Answer from the drawing. Dimensions are ordinates in mm from the lowest x, y and z of the part. A direction names the side the tool comes from. Give positions to 0.01 mm unless a question says otherwise; leave off trailing zeros. Loops run counter-clockwise (first coordinate to the right, second up) from the corner with the lowest first, then second, coordinate; pieces in that order, holes last.
(1) Each of these flat-tipped pins is pushed along its axis until it touches: P1, Ø4, axis at x = 43.5, z = 11.5, coming from the +Y side; P2, Ø5.5, axis at x = 30.5, z = 74.5, coming from the -Y side (3 decimals); P3, Ø5, axis at x = 28.5, y = 22, coming from the -Z side. Where does it stop, or does it pass through?
(2) Find section D-D, the plane y = 32. Write down the section's boundary in (x, z), then the cut area to 3 significant figures.
(3) Find section C-C, the plane x = 46.5. Write down the section's boundary in (y, z) (3 decimals).
(4) Determine the mould class of the marked faces 4, 5, 6 and 7 for opening direction Z: pulls with the +Z half, pulls with the -Z half, needs draft (parallel to the pull), parting line crosses it, or undercut.
(5) Which of the six approach directions +Z, -Z, +X, -X, +Y, -Y give full straight-line access (tool end or side, diameter ignored) to the marked faces 1, 2 and 3?
(6) Find section A-A, the plane y = 10. Write down the section's boundary in (x, z).
(7) Find section B-B, the plane z = 17. Write down the section's boundary in (x, y), then the cut area to 3 significant figures.
(8) Straight lines are drawn through the part: probe 1 along Z at (x, y) = (48.5, 12); probe 2 along Z at (x, y) = (14, 10.5); probe 3 along Y at (x, z) = (30, 67) (3 decimals). For each, find the intervals that lie inside material, in ascending order.
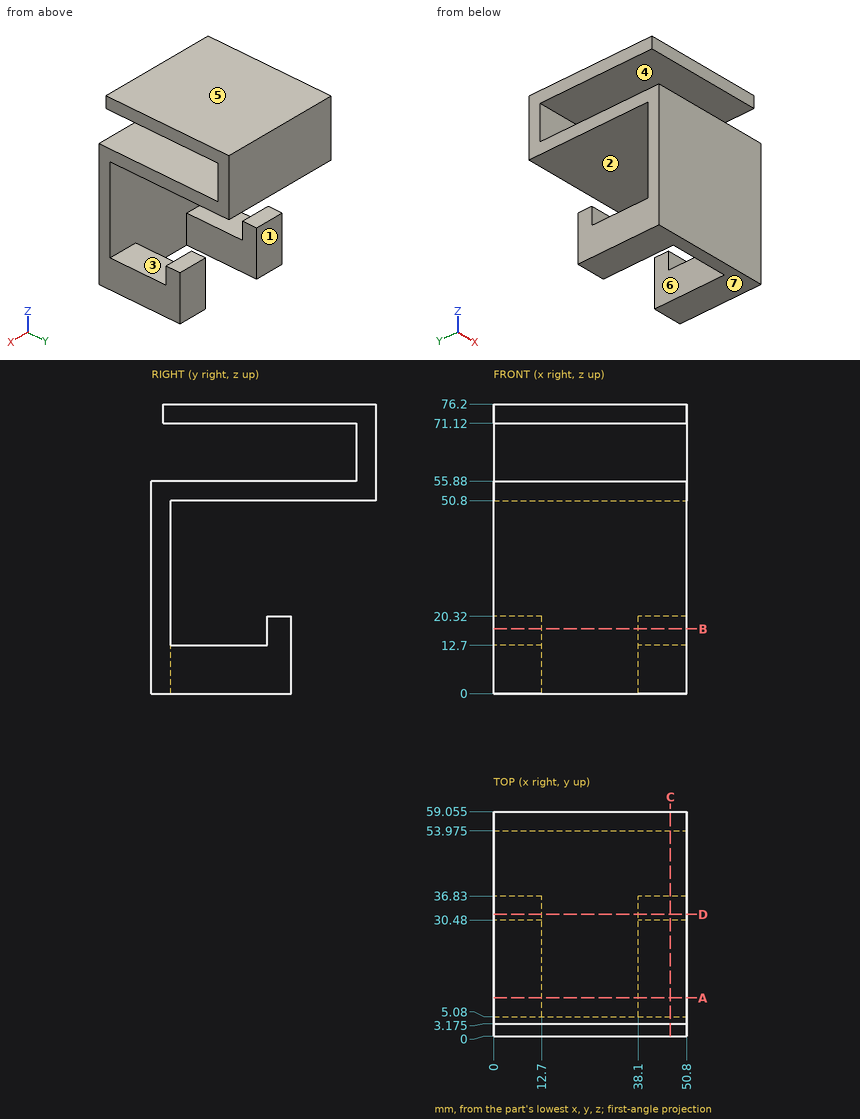
Entries:
1. P1: stops at y = 36.83
1. P2: stops at y = 3.175
1. P3: stops at z = 50.8
2. outline: (0, 0) - (12.7, 0) - (12.7, 20.32) - (0, 20.32) - close; (0, 50.8) - (50.8, 50.8) - (50.8, 55.88) - (0, 55.88) - close; (0, 71.12) - (50.8, 71.12) - (50.8, 76.2) - (0, 76.2) - close; (38.1, 0) - (50.8, 0) - (50.8, 20.32) - (38.1, 20.32) - close
2. area: 1,030 mm2
3. outline: (0, 0) - (36.83, 0) - (36.83, 20.32) - (30.48, 20.32) - (30.48, 12.7) - (5.08, 12.7) - (5.08, 50.8) - (59.055, 50.8) - (59.055, 76.2) - (3.175, 76.2) - (3.175, 71.12) - (53.975, 71.12) - (53.975, 55.88) - (0, 55.88) - close
4. face 4: undercut
4. face 5: pulls with the +Z half
4. face 6: needs draft
4. face 7: pulls with the -Z half
5. face 1: -Z, +X, -X, +Y
5. face 2: +X, -X, +Y
5. face 3: +X, -X
6. outline: (0, 0) - (12.7, 0) - (12.7, 12.7) - (0, 12.7) - close; (0, 50.8) - (50.8, 50.8) - (50.8, 55.88) - (0, 55.88) - close; (0, 71.12) - (50.8, 71.12) - (50.8, 76.2) - (0, 76.2) - close; (38.1, 0) - (50.8, 0) - (50.8, 12.7) - (38.1, 12.7) - close
7. outline: (0, 0) - (50.8, 0) - (50.8, 5.08) - (0, 5.08) - close; (0, 30.48) - (12.7, 30.48) - (12.7, 36.83) - (0, 36.83) - close; (38.1, 30.48) - (50.8, 30.48) - (50.8, 36.83) - (38.1, 36.83) - close
7. area: 419 mm2
8. probe 1: z = 0 to 12.7, 50.8 to 55.88, 71.12 to 76.2
8. probe 2: z = 50.8 to 55.88, 71.12 to 76.2
8. probe 3: y = 53.975 to 59.055
